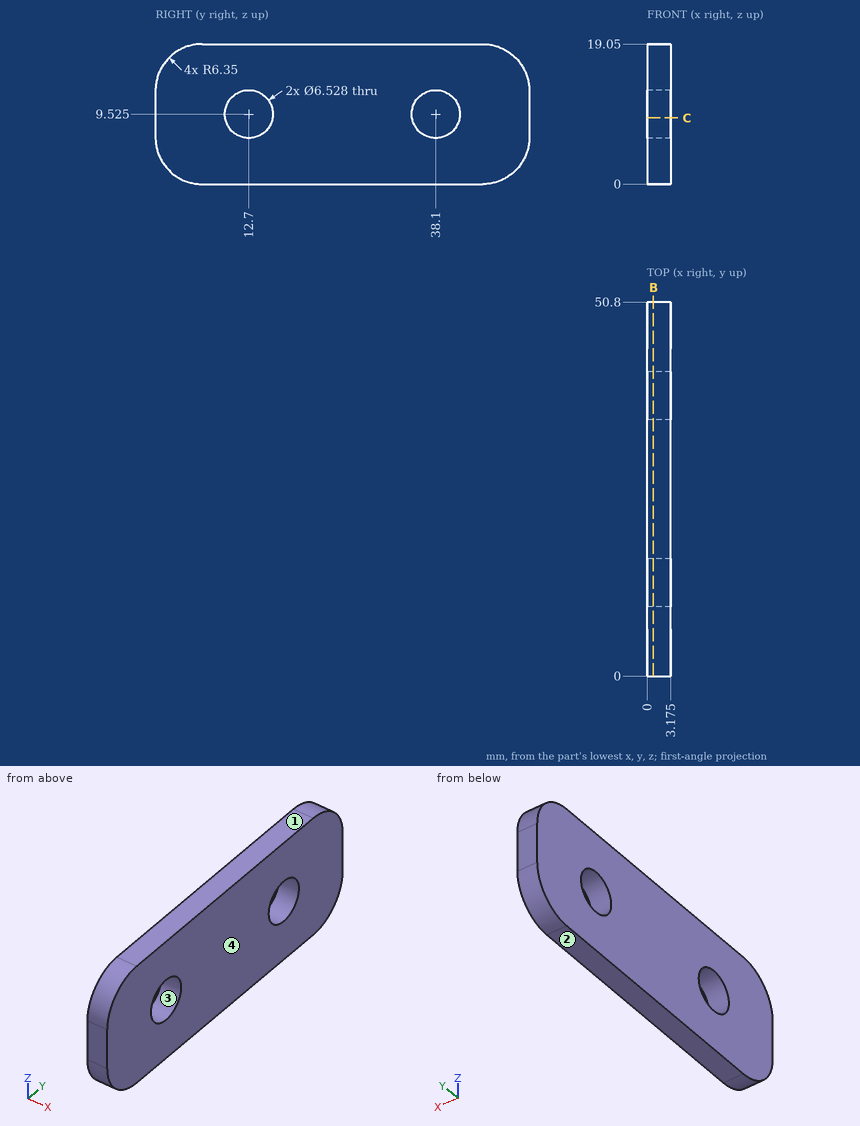
Here's the drawing with two shaded views (mm, measured from the low corner). I have some questions. Give positions to 0.01 mm unless a question says otherwise; leave off trailing zeros. Write each loop counter-clockwise with the first axis right and the second up, starting at its lowest first coordinate (ties: lowest second). Pieces come first, ordered by that corner, then holes. Notation, with made-up numbers: (-38, -35.5) -> (11, -35.5) arc R12 ccw to (11, -26.5) -> close; hole circle Ø7 at (19, 72). An arc over 180 degrees is marked (long way). Use one line per item in the form item = value.
1) We'd pull the mould along Z, two halves only. Please class the marked faces 1, 2, 3 and 4: +Z half, -Z half, draft (parallel to the pull), parting line (faces both ways), or undercut.
Verdict:
face_1 = +Z half
face_2 = -Z half
face_3 = undercut
face_4 = draft
2) Suppose I cut it at B-B (x = 0.85). Give the number of separate pieces and of enclosed holes in the cut face, and give its area (3 significant figures).
Verdict:
separate_pieces = 1
enclosed_holes = 2
area = 866 mm2
3) Suppose I cut it at C-C (z = 9). Please give me the cut outline in (x, y) (1 decimal), and give its area (3 significant figures).
Verdict:
outline = (0, 0) -> (3.2, 0) -> (3.2, 9.5) -> (0, 9.5) -> close; (0, 15.9) -> (3.2, 15.9) -> (3.2, 34.9) -> (0, 34.9) -> close; (0, 41.3) -> (3.2, 41.3) -> (3.2, 50.8) -> (0, 50.8) -> close
area = 120 mm2
4) If I drill on L1, parallel to Y at x = 1.25, z = 9.5; L2, parallel to Y at x = 0.6, z = 12.5; L3, parallel to Y at x = 0.4, z = 6, over which ranges is the centre line in solid material (lowest first)? Write a range as [from, to].
Verdict:
L1 = [0, 9.44], [15.96, 34.84], [41.36, 50.8]
L2 = [0, 11.36], [14.04, 36.76], [39.44, 50.8]
L3 = [0.01, 50.79]
